Geometry: final body of the model. Coordinates: model frame, mm. Face numbers are marked on the shaded views. A direction names the side the tool comes from. Round coordinates to 2 decimals unless told otherwise and drop trailing zeros. Write each loop counter-clockwise with the first axis right and the second up, starting at its lowest first coordinate (ties: lowest second). Pieces come first, ordered by that corner, then holes. Notation, with made-up numbers: (-28.5, 15.5) -> (-1.5, 15.5) arc R33 cw to (-1.5, 50.5) -> close; hole circle Ø7 at (12.25, 18.5). An arc over 180 degrees is marked (long way). Use one line per item in the form item = value. Start each with the question number.
1. Line query: L1, parallel to Z at x = -10.5, y = 5; L2, parallel to Z at x = -9, y = 2.75; L3, parallel to X at y = -1.5, z = 13.5. Output: solid intervals per line, ascending.
2. Cut plane D-D, the plane z = 13. Return the cut outline in (x, y).
3. Cut plane B-B, the plane z = 8. Return the cut outline in (x, y), plus the area to 3 significant figures.
4. Reachability of the marked faces 4, 5, 6, 7 and 8 from +Z, -Z, +X, -X, +Y, -Y: full face, straight path, thin tool, end or side. Return the list, or none.
5. Cut plane C-C, the plane y = -0.5. Return the cut outline in (x, z), plus the area to 3 significant figures.
6. Draft query along Z for the marked faces 1, 2 and 3. Return one class per face: pulls with the +Z half, pulls with the -Z half, needs draft (parallel to the pull), parting line crosses it, or undercut.
7. Pin query (flat end, axial travel): pin 1 Ø2 at (y, z) = (3, 10) entering from -X; pin 2 Ø6.5 at (x, y) = (-7.5, -4) entering from -Z; pin 3 Ø4.5 at (x, z) = (0.99, 9.48) entering from -Y; pin 4 Ø5 at (x, y) = (12.5, -3) entering from -Z. Return the tip coordinate at first contact, or that it passes through.
8. Cut plane A-A, the plane x = 6. Return the cut outline in (y, z).
```python
from build123d import *

# Parameters (mm, degrees)
SKETCH_1_W          = 7.5
SKETCH_1_H          = 6
EXTRUDE_1_DEPTH     = 3
EXTRUDE_2_DEPTH     = 6
SKETCH_3_R          = 2
CUT_EXTRUDE_1_DEPTH = 1
EXTRUDE_3_DEPTH     = 3.7
EXTRUDE_4_DEPTH     = 11.6
CUT_EXTRUDE_2_DEPTH = 12


with BuildPart() as part:
    # 草图1 → 凸台-拉伸1 (new body)
    with BuildSketch(Plane(origin=(0, 0, 0), x_dir=(1, 0, 0), z_dir=(0, 1, 0))):
        Polygon((23.991089217, -4.397070764), (23.991089217, -14.397070764), (16.47582205, -14.397070764), (16.47582205, -15.197070764), (2.97582205, -15.197070764), (-4.02417795, -15.197070764), (-16.008910783, -15.197070764), (-16.008910783, -3.597070764), (-4.02417795, -3.597070764), (2.97582205, -3.597070764), (16.47582205, -3.597070764), (16.47582205, -4.397070764), align=None)
        with Locations((-9.258910783, -9.397070764)):
            Rectangle(SKETCH_1_W, SKETCH_1_H, mode=Mode.SUBTRACT)
    extrude(amount=EXTRUDE_1_DEPTH)

    # 草图2 → 凸台-拉伸2 (add)
    with BuildSketch(Plane.XZ):
        Polygon((-13.008910783, 12.397070764), (-13.008910783, 13.897070764), (-3.008910783, 13.897070764), (-3.008910783, 4.897070764), (-13.008910783, 4.897070764), (-13.008910783, 6.397070764), (-5.508910783, 6.397070764), (-5.508910783, 12.397070764), align=None)
    extrude(amount=EXTRUDE_2_DEPTH)

    # 草图3 → 切除-拉伸1 (cut)
    with BuildSketch(Plane(origin=(0, 3, 0), x_dir=(1, 0, 0), z_dir=(0, 1, 0))):
        with Locations(Location((0.991089217, -9.484524381, 0), (0, 0, 270))):
            Circle(SKETCH_3_R)
    extrude(amount=-CUT_EXTRUDE_1_DEPTH, mode=Mode.SUBTRACT)

    # 草图4 → 凸台-拉伸3 (add)
    with BuildSketch(Plane(origin=(0, 3, 0), x_dir=(1, 0, 0), z_dir=(0, 1, 0))):
        Polygon((-16.008910783, -3.597070764), (13.47582205, -3.597070764), (13.47582205, -4.397070764), (-15.008910783, -4.397070764), (-15.008910783, -14.397070764), (13.47582205, -14.397070764), (13.47582205, -15.197070764), (-16.008910783, -15.197070764), align=None)
    extrude(amount=EXTRUDE_3_DEPTH)

    # 草图7 → 凸台-拉伸4 (add)
    with BuildSketch(Plane.XY.offset(15.197070764)):
        Polygon((-16.008910783, 0), (-16.008910783, 6.7), (-18.447511353, 0), align=None)
    extrude(amount=-EXTRUDE_4_DEPTH)

    # 草图8 → 切除-拉伸2 (cut)
    with BuildSketch(Plane.XY.offset(15.197070764)):
        Polygon((-16.008910783, 6.7), (-18.447511353, 0), (-17.926064244, 0), (-15.487463675, 6.7), align=None)
    extrude(amount=-CUT_EXTRUDE_2_DEPTH, mode=Mode.SUBTRACT)


solid = part.part
```
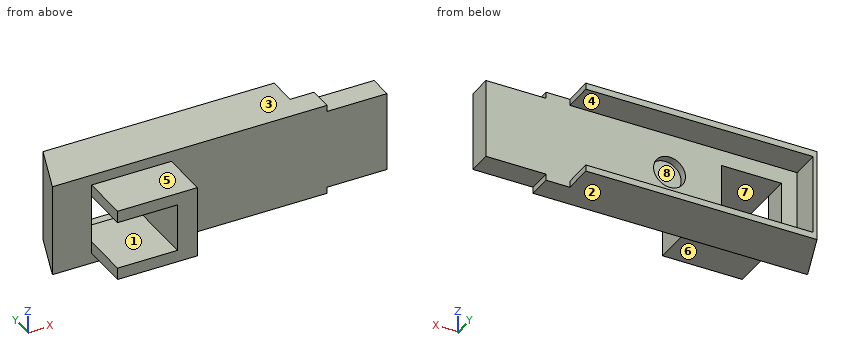
Outcome:
q1.L1 = 3.6 to 4.4, 14.4 to 15.2
q1.L2 = 3.6 to 6.4, 12.4 to 15.2
q1.L3 = -13.01 to -3.01
q2.outline = (-17.93, 0) -> (-13.01, 0) -> (-13.01, -6) -> (-3.01, -6) -> (-3.01, 0) -> (23.99, 0) -> (23.99, 3) -> (-15.01, 3) -> (-15.01, 6.7) -> (-15.49, 6.7) -> close
q3.outline = (-17.93, 0) -> (-13.01, 0) -> (-13.01, 3) -> (-15.01, 3) -> (-15.01, 6.7) -> (-15.49, 6.7) -> close; (-5.51, -6) -> (-3.01, -6) -> (-3.01, 0) -> (23.99, 0) -> (23.99, 3) -> (2.33, 3) -> (2.33, 2) -> (-0.35, 2) -> (-0.35, 3) -> (-5.51, 3) -> close
q3.area = 118 mm^2
q4.face_4 = +X, +Y
q4.face_5 = +Z, +X, -X, -Y
q4.face_6 = -Z, +X, -X, -Y
q4.face_7 = +Y, -Y
q4.face_8 = +Y
q5.outline = (-13.01, 4.9) -> (-3.01, 4.9) -> (-3.01, 13.9) -> (-13.01, 13.9) -> (-13.01, 12.4) -> (-5.51, 12.4) -> (-5.51, 6.4) -> (-13.01, 6.4) -> close
q5.area = 45.0 mm^2
q6.face_1 = undercut
q6.face_2 = pulls with the -Z half
q6.face_3 = pulls with the +Z half
q7.pin_1 = -17.2
q7.pin_2 = 4.9
q7.pin_3 = 0
q7.pin_4 = through
q8.outline = (0, 3.6) -> (6.7, 3.6) -> (6.7, 4.4) -> (3, 4.4) -> (3, 14.4) -> (6.7, 14.4) -> (6.7, 15.2) -> (0, 15.2) -> close
